from build123d import *

# Parameters (mm, degrees)
SKETCH2_R           = 18.85
SKETCH2_R_2         = 17
BOSS_EXTRUDE1_DEPTH = 2
SKETCH9_R           = 3.098061326
BOSS_EXTRUDE5_DEPTH = 2
BOSS_EXTRUDE2_START = -1
SKETCH3_R           = 35
SKETCH3_R_2         = 18.85
BOSS_EXTRUDE2_DEPTH = 1
SKETCH4_R           = 2.9
BOSS_EXTRUDE3_DEPTH = 3
SKETCH6_R           = 5
BOSS_EXTRUDE4_DEPTH = 1
SKETCH7_R           = 59.131365533
CUT_EXTRUDE1_DEPTH  = 10
FILLET1_R           = 6


with BuildPart() as part:
    # Sketch2 → Boss-Extrude1 (new body)
    # profile 1 of 10: a face of its own
    with BuildSketch(Plane.XY.offset(10)):
        Circle(SKETCH2_R)
        Circle(SKETCH2_R_2, mode=Mode.SUBTRACT)
    # profile 2 of 10: a face of its own
    with BuildSketch(Plane.XY.offset(10)):
        with BuildLine():
            ThreePointArc((-1.02606043, 2.819077862), (-0.520944533, 2.954423259), (0, 3))
            Line((0, 3), (0, 17))
            ThreePointArc((0, 17), (-2.95201902, 16.741731801), (-5.814342437, 15.974774553))
            Line((-5.814342437, 15.974774553), (-1.02606043, 2.819077862))
        make_face()
    # profile 3 of 10: a face of its own
    with BuildSketch(Plane.XY.offset(10)):
        with BuildLine():
            Line((5.814342437, 15.974774553), (1.02606043, 2.819077862))
            ThreePointArc((1.02606043, 2.819077862), (1.5, 2.598076211), (1.928362829, 2.298133329))
            Line((1.928362829, 2.298133329), (10.927389365, 13.022755533))
            ThreePointArc((10.927389365, 13.022755533), (8.5, 14.722431864), (5.814342437, 15.974774553))
        make_face()
    # profile 4 of 10: a face of its own
    with BuildSketch(Plane.XY.offset(10)):
        with BuildLine():
            Line((14.722431864, 8.5), (2.598076211, 1.5))
            ThreePointArc((2.598076211, 1.5), (2.819077862, 1.02606043), (2.954423259, 0.520944533))
            Line((2.954423259, 0.520944533), (16.741731801, 2.95201902))
            ThreePointArc((16.741731801, 2.95201902), (15.974774553, 5.814342437), (14.722431864, 8.5))
        make_face()
    # profile 5 of 10: a face of its own
    with BuildSketch(Plane.XY.offset(10)):
        with BuildLine():
            Line((16.741731801, -2.95201902), (2.954423259, -0.520944533))
            ThreePointArc((2.954423259, -0.520944533), (2.819077862, -1.02606043), (2.598076211, -1.5))
            Line((2.598076211, -1.5), (14.722431864, -8.5))
            ThreePointArc((14.722431864, -8.5), (15.974774553, -5.814342437), (16.741731801, -2.95201902))
        make_face()
    # profile 6 of 10: a face of its own
    with BuildSketch(Plane.XY.offset(10)):
        with BuildLine():
            Line((10.927389365, -13.022755533), (1.928362829, -2.298133329))
            ThreePointArc((1.928362829, -2.298133329), (1.5, -2.598076211), (1.02606043, -2.819077862))
            Line((1.02606043, -2.819077862), (5.814342437, -15.974774553))
            ThreePointArc((5.814342437, -15.974774553), (8.5, -14.722431864), (10.927389365, -13.022755533))
        make_face()
    # profile 7 of 10: a face of its own
    with BuildSketch(Plane.XY.offset(10)):
        with BuildLine():
            ThreePointArc((0, -3), (-0.520944533, -2.954423259), (-1.02606043, -2.819077862))
            Line((-1.02606043, -2.819077862), (-5.814342437, -15.974774553))
            ThreePointArc((-5.814342437, -15.974774553), (-2.95201902, -16.741731801), (0, -17))
            Line((0, -17), (0, -3))
        make_face()
    # profile 8 of 10: a face of its own
    with BuildSketch(Plane.XY.offset(10)):
        with BuildLine():
            ThreePointArc((-1.928362829, -2.298133329), (-2.298133329, -1.928362829), (-2.598076211, -1.5))
            Line((-2.598076211, -1.5), (-14.722431864, -8.5))
            ThreePointArc((-14.722431864, -8.5), (-13.022755533, -10.927389365), (-10.927389365, -13.022755533))
            Line((-10.927389365, -13.022755533), (-1.928362829, -2.298133329))
        make_face()
    # profile 9 of 10: a face of its own
    with BuildSketch(Plane.XY.offset(10)):
        with BuildLine():
            ThreePointArc((-2.954423259, -0.520944533), (-3, 0), (-2.954423259, 0.520944533))
            Line((-2.954423259, 0.520944533), (-16.741731801, 2.95201902))
            ThreePointArc((-16.741731801, 2.95201902), (-17, 0), (-16.741731801, -2.95201902))
            Line((-16.741731801, -2.95201902), (-2.954423259, -0.520944533))
        make_face()
    # profile 10 of 10: a face of its own
    with BuildSketch(Plane.XY.offset(10)):
        with BuildLine():
            ThreePointArc((-2.598076211, 1.5), (-2.298133329, 1.928362829), (-1.928362829, 2.298133329))
            Line((-1.928362829, 2.298133329), (-10.927389365, 13.022755533))
            ThreePointArc((-10.927389365, 13.022755533), (-13.022755533, 10.927389365), (-14.722431864, 8.5))
            Line((-14.722431864, 8.5), (-2.598076211, 1.5))
        make_face()
    extrude(amount=-BOSS_EXTRUDE1_DEPTH)

    # Sketch9 → Boss-Extrude5 (add)
    with BuildSketch(Plane.XY.offset(10)):
        Circle(SKETCH9_R)
    extrude(amount=-BOSS_EXTRUDE5_DEPTH)

    # Sketch3 → Boss-Extrude2 (add)
    with BuildSketch(Plane(origin=(0, 0, 8), x_dir=(-1, 0, 0), z_dir=(0, 0, -1)).offset(BOSS_EXTRUDE2_START)):
        Circle(SKETCH3_R)
        with Locations(Location((0, 0, 0), (0, 0, 180))):
            Circle(SKETCH3_R_2, mode=Mode.SUBTRACT)
    extrude(amount=BOSS_EXTRUDE2_DEPTH)

    # Sketch4 → Boss-Extrude3 (add)
    with BuildSketch(Plane(origin=(0, 0, 8), x_dir=(-1, 0, 0), z_dir=(0, 0, -1))):
        with Locations((0, 29)):
            Circle(SKETCH4_R)
        with Locations((25.11473671, -14.5)):
            Circle(SKETCH4_R)
        with Locations((-25.11473671, -14.5)):
            Circle(SKETCH4_R)
    extrude(amount=-BOSS_EXTRUDE3_DEPTH)

    # Sketch6 → Boss-Extrude4 (add)
    with BuildSketch(Plane(origin=(0, 0, 9), x_dir=(-1, 0, 0), z_dir=(0, 0, -1))):
        with Locations((0, 30)):
            Circle(SKETCH6_R)
        with Locations((25.980762114, -15)):
            Circle(SKETCH6_R)
        with Locations((-25.980762114, -15)):
            Circle(SKETCH6_R)
    extrude(amount=BOSS_EXTRUDE4_DEPTH)

    # Sketch7 → Cut-Extrude1 (cut)
    with BuildSketch(Plane(origin=(0, 0, 8), x_dir=(-1, 0, 0), z_dir=(0, 0, -1))):
        Circle(SKETCH7_R)
        Polygon((0, 42), (-36.373066959, -21), (36.373066959, -21), align=None, mode=Mode.SUBTRACT)
    extrude(amount=-CUT_EXTRUDE1_DEPTH, mode=Mode.SUBTRACT)

    # Fillet1
    fillet1_edges = [part.edges().sort_by_distance(p)[0] for p in [
        (-4.186533479, 34.748711306, 8.5),
        (-32.186533479, -13.748711306, 8.5),
        (-28, -21, 8.5),
        (28, -21, 8.5),
        (32.186533479, -13.748711306, 8.5),
        (4.186533479, 34.748711306, 8.5),
    ]]
    fillet(fillet1_edges, radius=FILLET1_R)


solid = part.part
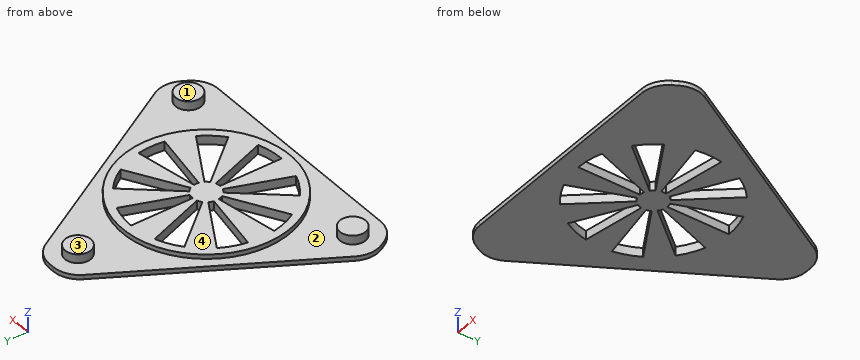
Work out the finished part from the listing and answer in its coordinate system (mm). Face numbers are marked on the shaded views. A direction names the side the tool comes from. Round coordinates to 2 decimals unless told otherwise and drop trailing zeros. Write each loop counter-clockwise with the first axis right and the second up, starting at its lowest first coordinate (ties: lowest second). Pieces come first, ordered by that corner, then holes.
1) A tool of negligible diameter and unlimited length cuts with its end or side. For the marked faces 1 and 2, from which of +Z, -Z, +X, -X, +Y, -Y can it reach the whole face along a straight path? Write none if from no direction.
2) A cutting plane is placed at D-D (y = 27.5). Give the vertices of the cut face in (x, z).
3) A cutting plane is placed at B-B (y = -7.5). Give the vertices of the cut face in (x, z), plus the area to 3 significant figures.
4) Given pin 1 Ø11.5 at (x, y) = (3.5, -4.5) entering from +Z; pin 2 Ø1.6 at (y, z) = (-7.5, 9.5) entering from +X; pin 3 Ø0.6 at (y, z) = (9, 9.5) entering from +X; pin 4 Ø6 at (x, y) = (-20, 19) entering from +Z, each flat-ended and moving along its own axis, determine where each tip first touches the part or whether it passes through.
5) A cutting plane is placed at A-A (x = -4). Give the vertices of the cut face in (y, z).
6) The mould has two halves that part along X. Classify the marked faces 3 and 4: pulls with the +X half, pulls with the -X half, needs draft (parallel to the pull), parting line crosses it, or undercut.
7) Straight lines are drawn through the part: line 1 (X direction, y = 7, z = 8.15); line 2 (Y direction, x = -14.5, z = 9.8); line 3 (Y direction, x = -15, z = 8.9). For each, find the intervals that lie inside material, in ascending order.
8) A cutting plane is placed at C-C (y = -14.5). Give the vertices of the cut face in (x, z), plus the area to 3 significant figures.
Completed:
1. face 1: +Z, +X, -X, +Y, -Y
1. face 2: +Z
2. outline: (-8.37, 8) - (8.37, 8) - (8.37, 9) - (2.48, 9) - (2.48, 11) - (-2.48, 11) - (-2.48, 9) - (-8.37, 9) - close
3. outline: (-28.58, 8) - (-15.26, 8) - (-15.26, 10) - (-17.29, 10) - (-17.29, 9) - (-28.58, 9) - close; (-12.99, 8) - (-6.29, 8) - (-6.29, 10) - (-12.99, 10) - close; (-2.73, 8) - (0, 8) - (0, 10) - (-2.73, 10) - close; (2.73, 8) - (6.29, 8) - (6.29, 10) - (2.73, 10) - close; (12.99, 8) - (28.58, 8) - (28.58, 9) - (17.29, 9) - (17.29, 10) - (12.99, 10) - close
3. area: 61.2 mm2
4. pin 1: stops at z = 10
4. pin 2: stops at x = 28.94
4. pin 3: stops at x = 16.72
4. pin 4: passes through
5. outline: (-21, 8) - (-10.99, 8) - (-10.99, 10) - (-18.42, 10) - (-18.42, 9) - (-21, 9) - close; (-4.77, 8) - (-2.31, 8) - (-2.31, 10) - (-4.77, 10) - close; (-0.71, 8) - (0.71, 8) - (0.71, 10) - (-0.71, 10) - close; (2.31, 8) - (4.77, 8) - (4.77, 10) - (2.31, 10) - close; (10.99, 8) - (33.92, 8) - (33.92, 9) - (18.42, 9) - (18.42, 10) - (10.99, 10) - close
6. face 3: needs draft
6. face 4: undercut
7. line 1: x = -20.21 to -15.49, -12.12 to -5.87, -2.55 to 0, 2.55 to 5.87, 12.12 to 20.21
7. line 2: y = -12.04 to -8.37, -2.56 to 2.56, 8.37 to 12.04
7. line 3: y = -21 to -8, -2.64 to 2.64, 8 to 16.02
8. outline: (-31.38, 8) - (-8.87, 8) - (-8.87, 10) - (-12.04, 10) - (-12.04, 9) - (-22.21, 9) - (-22.21, 11) - (-28.01, 11) - (-28.01, 9) - (-31.38, 9) - close; (-5.28, 8) - (0, 8) - (0, 10) - (-5.28, 10) - close; (5.28, 8) - (31.38, 8) - (31.38, 9) - (28.01, 9) - (28.01, 11) - (22.21, 11) - (22.21, 9) - (12.04, 9) - (12.04, 10) - (5.28, 10) - close
8. area: 92.3 mm2
